The model under review builds one solid part; all positions refer to its coordinate system, in mm. A direction names the side the tool comes from. Give positions to 0.01 mm unless a question says otherwise; leave off trailing zeros. Order: outer loops, then holes, each group sorted by start corner. A loop starts at its lowest first (then second) coordinate and runs counter-clockwise, first axis right, second up. Notation, with made-up numbers: (10.5, -17.5) - (46.5, -17.5) arc R17 cw to (46.5, 13.5) - close; hole circle Ø11 at (22.25, -27.5). An arc over 180 degrees is marked (long way). Put each result on its own line as item: value.
```python
from build123d import *

# Parameters (mm, degrees)
SKETCH1_R                = 1.3589
BOSS_EXTRUDE1_DEPTH      = 2.2352
SKETCH2_R                = 5.334
BOSS_EXTRUDE2_DEPTH      = 7.2136
BOSS_EXTRUDE3_DEPTH      = 7.9121
BOSS_EXTRUDE3_DEPTH_BACK = 7.9121
SKETCH3_R                = 1.4732
SKETCH4_R                = 3.96875
BOSS_EXTRUDE4_DEPTH      = 8.2042
SKETCH5_R                = 16.51
BOSS_EXTRUDE5_DEPTH      = 11.684
SKETCH6_R                = 3.4925
BOSS_EXTRUDE6_DEPTH      = 5.3594
SKETCH7_R                = 1.4859
BOSS_EXTRUDE7_DEPTH      = 8.5852


with BuildPart() as part:
    # Sketch1 → Boss-Extrude1 (new body)
    with BuildSketch(Plane.XY):
        with BuildLine():
            ThreePointArc((2.2987, -7.9248), (4.217475252, -3.616655942), (8.703337155, -2.161030069))
            ThreePointArc((8.703337155, -2.161030069), (9.097483524, -2.216404696), (9.4869, -2.2987))
            ThreePointArc((9.4869, -2.2987), (11.7856, 0), (9.4869, 2.2987))
            ThreePointArc((9.4869, 2.2987), (4.922822315, 3.872455712), (2.2987, 7.9248))
            ThreePointArc((2.2987, 7.9248), (0, 10.2235), (-2.2987, 7.9248))
            ThreePointArc((-2.2987, 7.9248), (-4.217475252, 3.616655942), (-8.703337155, 2.161030069))
            ThreePointArc((-8.703337155, 2.161030069), (-9.097483524, 2.216404696), (-9.4869, 2.2987))
            ThreePointArc((-9.4869, 2.2987), (-11.7856, 0), (-9.4869, -2.2987))
            ThreePointArc((-9.4869, -2.2987), (-4.922822315, -3.872455712), (-2.2987, -7.9248))
            ThreePointArc((-2.2987, -7.9248), (0, -10.2235), (2.2987, -7.9248))
        make_face()
        with Locations((0, -7.9248)):
            Circle(SKETCH1_R, mode=Mode.SUBTRACT)
        with Locations((-9.4869, 0)):
            Circle(SKETCH1_R, mode=Mode.SUBTRACT)
        with Locations((0, 7.9248)):
            Circle(SKETCH1_R, mode=Mode.SUBTRACT)
        with Locations((9.4869, 0)):
            Circle(SKETCH1_R, mode=Mode.SUBTRACT)
    extrude(amount=BOSS_EXTRUDE1_DEPTH)

    # Sketch2 → Boss-Extrude2 (add)
    with BuildSketch(Plane.XY.offset(2.2352)):
        Circle(SKETCH2_R)
    extrude(amount=BOSS_EXTRUDE2_DEPTH)

    # Sketch3 → Boss-Extrude3 (add, two sides: drawn at the far end of the back side and taken through both)
    with BuildSketch(Plane(origin=(0, 0, 0), x_dir=(0, 0, -1), z_dir=(1, 0, 0)).offset(-BOSS_EXTRUDE3_DEPTH_BACK)):
        with Locations((-6.6548, 0)):
            Circle(SKETCH3_R)
    extrude(amount=BOSS_EXTRUDE3_DEPTH + BOSS_EXTRUDE3_DEPTH_BACK)

    # Sketch4 → Boss-Extrude4 (add)
    with BuildSketch(Plane.XY.offset(9.4488)):
        Circle(SKETCH4_R)
    extrude(amount=BOSS_EXTRUDE4_DEPTH)

    # Sketch5 → Boss-Extrude5 (add)
    with BuildSketch(Plane.XY.offset(17.653)):
        Circle(SKETCH5_R)
    extrude(amount=BOSS_EXTRUDE5_DEPTH)

    # Sketch6 → Boss-Extrude6 (add)
    with BuildSketch(Plane.XY.offset(29.337)):
        Circle(SKETCH6_R)
    extrude(amount=BOSS_EXTRUDE6_DEPTH)

    # Sketch7 → Boss-Extrude7 (add)
    with BuildSketch(Plane.XY.offset(34.6964)):
        Circle(SKETCH7_R)
    extrude(amount=BOSS_EXTRUDE7_DEPTH)


solid = part.part
```
(1) For faces 1 (the cylindrical face through (-0.295, -9.251, 1.102)), 2 (the cylindrical face through (4.98, 3.83, 1.1)), 3 (the cylindrical face through (-0.051, -10.223, 1.102)), list the 3-axis set-ups (+Z, -Z, +X, -X, +Y, -Y) from which the entire face can be reached by the end or side of a thin tool; tool diameter is ignored.
The answers:
face 1: -Z
face 2: -Z, +X, +Y
face 3: -Z, -Y
(2) Take a section at C-C, the plane x = 6. Write out the cut boundary in (y, z), then the cut area to 3 significant figures.
The answers:
outline: (-15.38, 17.65) - (15.38, 17.65) - (15.38, 29.34) - (-15.38, 29.34) - close; (-2.52, 0) - (3.17, 0) - (3.17, 2.24) - (-2.52, 2.24) - close; circle Ø2.95 at (0, 6.65)
area: 379 mm^2
(3) Clearance check with flat-ended pins moving along their axes: pin 1 Ø12 at (x, z) = (-12.5, 24.5) entering from -Y; pin 2 Ø1.6 at (x, y) = (9.49, 0) entering from +Z; pin 3 Ø0.9 at (y, z) = (-0.5, 7.5) entering from +X; pin 4 Ø1.5 at (y, z) = (12, 15.5) entering from -X (3 decimals). State where each tip first meets the part, or that it passes through.
The answers:
pin 1: y = -15.18
pin 2: z = 29.34
pin 3: x = 7.91
pin 4: through
(4) Wall thickness on L1, parallel to Y at x = 0, z = 1.4; L2, parallel to Z at x = 2, y = -3.5; L3, parallel to Z at x = -9, y = -9: over which ranges is each line inside the solid? List them lowest first.
The answers:
L1: -10.22 to -9.28, -6.57 to 6.57, 9.28 to 10.22
L2: 0 to 9.45, 17.65 to 29.34
L3: 17.65 to 29.34
(5) Take a section at A-A, the plane x = 0. Count the separate pieces of the cut face and the enclosed holes in it, then the cut area to 3 significant figures.
The answers:
separate pieces: 3
enclosed holes: 0
area: 624 mm^2
(6) Take a section at D-D, the plane z = 35.5. Write out the cut boundary in (x, y).
The answers:
outline: circle Ø2.97 at (0, 0)
(7) The part is to be moulded in two halves that separate along Z. For faces 4 (the cylindrical face through (-10.488, 0.918, 1.102)), 5 (the cylindrical face through (4.93, -2.04, 5.79)), 6 (the flat face through (1, -1, 0)), say which applies: pulls with the +Z half, pulls with the -Z half, needs draft (parallel to the pull), parting line crosses it, or undercut.
The answers:
face 4: needs draft
face 5: undercut
face 6: pulls with the -Z half
